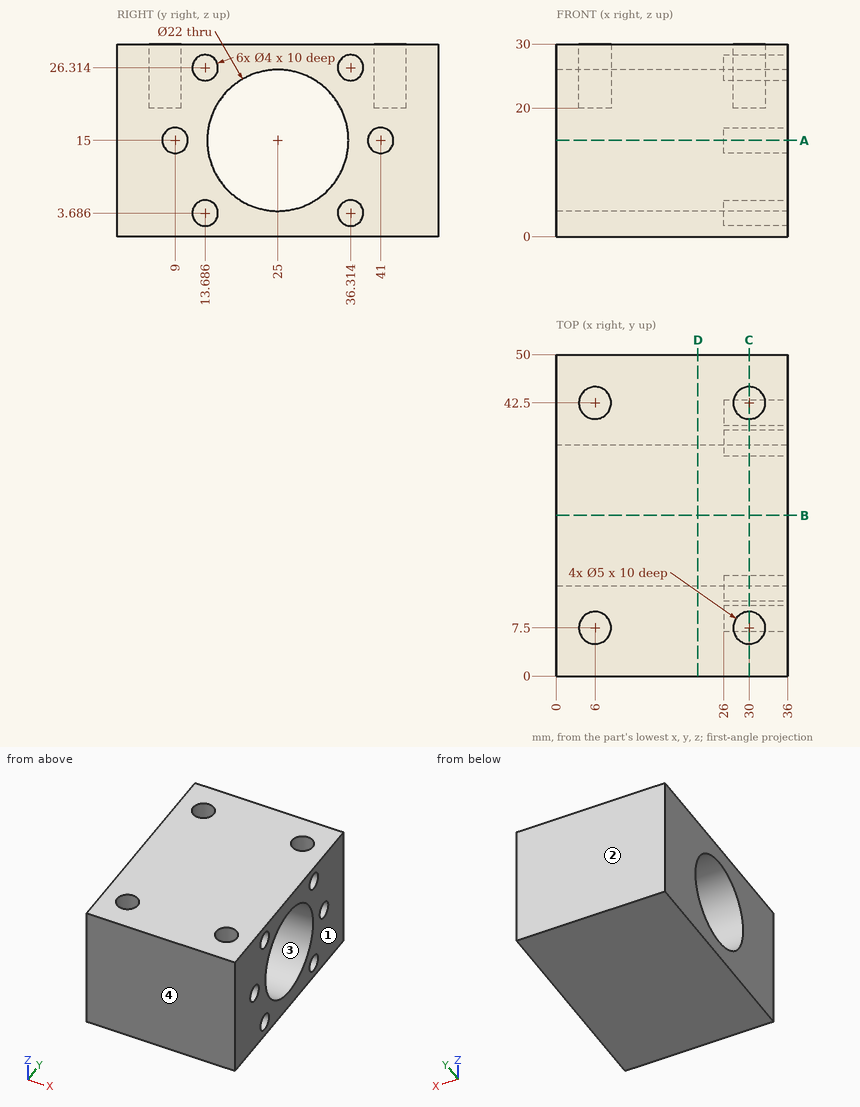
Geometry check sheet. Reference: drawing and pictorial views, mm from the part's lowest x, y, z. Round coordinates to 2 decimals unless told otherwise and drop trailing zeros. Order: outer loops, then holes, each group sorted by start corner. A loop starts at its lowest first (then second) coordinate and runs counter-clockwise, first axis right, second up.
Q1. Cross-section at D-D, the plane x = 22. Enter the section's corners in (y, z), plus the area to 3 significant figures.
Filled sheet:
outline: (0, 0) - (50, 0) - (50, 30) - (0, 30) - close; hole circle Ø22 at (25, 15)
area: 1,120 mm2
Q2. Draft check along Y on the marked faces 1, 2, 3 and 4. Enter one of: pulls with the +Y half, pulls with the -Y half, needs draft (parallel to the pull), parting line crosses it, or undercut.
Filled sheet:
face 1: needs draft
face 2: pulls with the +Y half
face 3: undercut
face 4: pulls with the -Y half
Q3. Cross-section at B-B, the plane y = 25. Enter the section's corners in (x, z).
Filled sheet:
outline: (0, 0) - (36, 0) - (36, 4) - (0, 4) - close; (0, 26) - (36, 26) - (36, 30) - (0, 30) - close
Q4. Depth check by flat-ended pin: P1, Ø3, axis at x = 30, y = 7.5, coming from the +Z side; P2, Ø2, axis at y = 9.5, z = 15, coming from the +X side. Enter the tip coordinate at first touch or a pass-through.
Filled sheet:
P1: stops at z = 20
P2: stops at x = 26
Q5. Cross-section at A-A, the plane z = 15. Enter the section's corners in (x, y), plus the area to 3 significant figures.
Filled sheet:
outline: (0, 0) - (36, 0) - (36, 7) - (26, 7) - (26, 11) - (36, 11) - (36, 14) - (0, 14) - close; (0, 36) - (36, 36) - (36, 39) - (26, 39) - (26, 43) - (36, 43) - (36, 50) - (0, 50) - close
area: 928 mm2
Q6. Scan lines: L1, parallel to Y at x = 6, z = 27.75; L2, parallel to Y at x = 30, z = 23.5; L3, parallel to Y at x = 13.5, z = 13. Record each from-to range of solid material in increasing order.
Filled sheet:
L1: y = 0 to 5, 10 to 40, 45 to 50
L2: y = 0 to 5, 10 to 18.02, 31.98 to 40, 45 to 50
L3: y = 0 to 14.18, 35.82 to 50
Q7. Cross-section at C-C, the plane x = 30. Enter the section's corners in (y, z).
Filled sheet:
outline: (0, 0) - (50, 0) - (50, 30) - (45, 30) - (45, 20) - (40, 20) - (40, 30) - (10, 30) - (10, 20) - (5, 20) - (5, 30) - (0, 30) - close; hole circle Ø4 at (9, 15); hole circle Ø4 at (13.69, 3.69); hole circle Ø4 at (13.69, 26.31); hole circle Ø22 at (25, 15); hole circle Ø4 at (36.31, 3.69); hole circle Ø4 at (36.31, 26.31); hole circle Ø4 at (41, 15)
